Answer from the drawing. Dimensions are ordinates in mm from the lowest x, y and z of the part. A direction names the side the tool comes from. Give positions to 0.01 mm unless a question says otherwise; leave off trailing zeros. Order: outer loops, then holes, each group sorted by start corner. A loop starts at its lowest first (then second) coordinate and runs counter-clockwise, first axis right, second up.
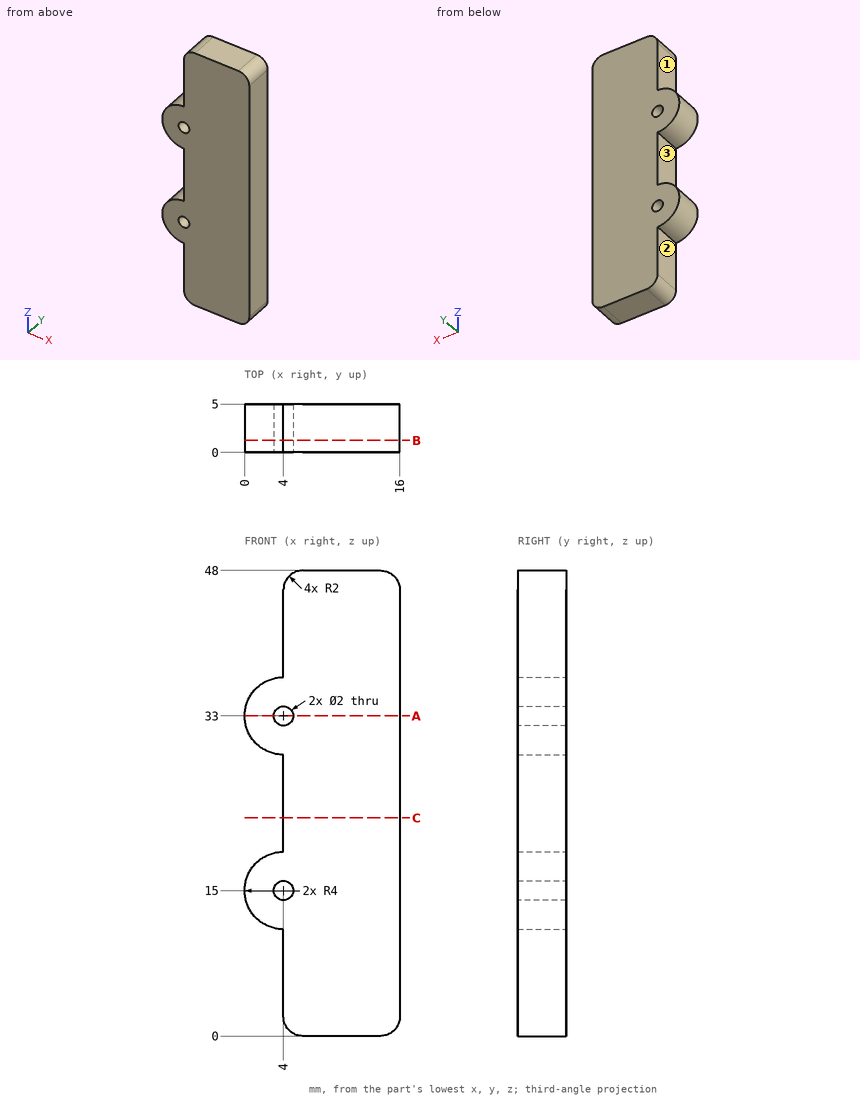
1. The part is cut by section A-A (z = 33). Write down the section's boundary in (x, y), then the cut area to 3 significant figures.
Findings below:
outline: (0, 0) - (3, 0) - (3, 5) - (0, 5) - close; (5, 0) - (16, 0) - (16, 5) - (5, 5) - close
area: 70.0 mm2
2. The part is cut by section C-C (z = 22.5). Write down the section's boundary in (x, y), then the cut area to 3 significant figures.
Findings below:
outline: (4, 0) - (16, 0) - (16, 5) - (4, 5) - close
area: 60.0 mm2
3. Given P1, Ø1.2, axis at x = 4, z = 15, coming from the +Y side; P2, Ø2, axis at x = 12, z = 20, coming from the -Y side; P3, Ø1, axis at x = 4.5, y = 0.5, coming from the +Z side; P4, Ø1.5, axis at y = 3.5, z = 8, coming from the -X side, each flat-ended and moving along its own axis, determine where each tip first touches the part or whether it passes through.
Findings below:
P1: passes through
P2: stops at y = 0
P3: stops at z = 47.73
P4: stops at x = 4
4. Straight lines are drawn through the part: probe 1 along X at (y, z) = (1.85, 33); probe 2 along X at (y, z) = (2.5, 45); probe 3 along Z at (x, y) = (2.75, 4.75). For each, find the intervals that lie inside material, in ascending order.
Findings below:
probe 1: x = 0 to 3, 5 to 16
probe 2: x = 4 to 16
probe 3: z = 11.2 to 18.8, 29.2 to 36.8
5. The part is cut by section B-B (y = 1.25). Write down the section's boundary in (x, z), then the cut area to 3 significant figures.
Findings below:
outline: (4, 2) arc R2 ccw to (6, 0) - (14, 0) arc R2 ccw to (16, 2) - (16, 46) arc R2 ccw to (14, 48) - (6, 48) arc R2 ccw to (4, 46) - (4, 37) arc R4 ccw to (4, 29) - (4, 19) arc R4 ccw to (4, 11) - close; hole circle Ø2 at (4, 15); hole circle Ø2 at (4, 33)
area: 617 mm2
6. Which of the six approach directions +Z, -Z, +X, -X, +Y, -Y give full straight-line access (tool end or side, diameter ignored) to the marked faces 1, 2 and 3?
Findings below:
face 1: +Z, -X, +Y, -Y
face 2: -Z, -X, +Y, -Y
face 3: -X, +Y, -Y
